from build123d import *

# Parameters (mm, degrees)
BOSS_EXTRUDE1_DEPTH = 25.4
CUT_EXTRUDE1_DEPTH  = 26.4


with BuildPart() as part:
    # Sketch1 → Boss-Extrude1 (new body)
    with BuildSketch(Plane.XY):
        Polygon((0, 0), (-6.35, 10.998522628), (-4.516912895, 10.998522628), (0.916543552, 1.5875), (14.958456448, 1.5875), (15.875, 0), align=None)
    extrude(amount=BOSS_EXTRUDE1_DEPTH)

    # Sketch2 → Cut-Extrude1 (cut, through all)
    with BuildSketch(Plane.XY.offset(25.4)):
        Polygon((-6.35, 10.998522628), (-2.79437447, 8.014998557), (-4.516912895, 10.998522628), align=None)
    extrude(amount=-CUT_EXTRUDE1_DEPTH, mode=Mode.SUBTRACT)


solid = part.part
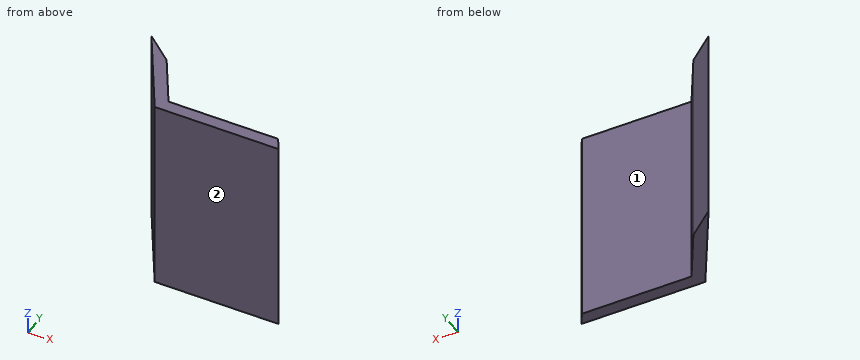
CAD build for the part. Positions are in the model's coordinates, mm. Face numbers are marked on the shaded views. A direction names the side the tool comes from. Give positions to 0.01 mm unless a question says otherwise; leave off trailing zeros. Order: outer loops, then holes, each group sorted by start corner. A loop starts at its lowest first (then second) coordinate and runs counter-clockwise, first axis right, second up. Notation, with made-up numbers: (24, 23) -> (60, 23) arc R15 cw to (60, 45) -> close; hole circle Ø11 at (29.25, 33). An arc over 180 degrees is marked (long way). Return JSON: item names as keys, results as strings.
Q1. Drill centre lines: line 1 (Y direction, x = 12.5, z = 15); line 2 (Y direction, x = -2.5, z = 13); line 3 (X direction, y = 8, z = 20.25). Where is each one in solid material? Low to high.
Working result:
{"line 1": "0 to 1.59", "line 2": "4.33 to 7.51", "line 3": "-4.62 to -2.79"}
Q2. Which spindle directions (+Z, -Z, +X, -X, +Y, -Y) get a long thin tool onto all of the face, cutting with end or side? Do the marked faces 1 and 2. Say none if no direction does.
Working result:
{"face 1": "+Z, -Z, +X, +Y", "face 2": "+Z, -Z, +X, -X, -Y"}
Q3. Flat gauge pins, fed straight in: pin 1 (3 mm diameter, centred on x = 8, z = 14, fed in from +Y); pin 2 (4 mm diameter, centred on y = 2, z = 21.5, fed in from -X); pin 3 (12 mm diameter, centred on x = 1.5, z = 6.5, fed in from +Y). Where does each tip first touch, or does it go through?
Working result:
{"pin 1": "y = 1.59", "pin 2": "x = -2.31", "pin 3": "y = 9.45"}
Q4. Saw through at C-C (y = 6). Write the cut outline in (x, z).
Working result:
{"outline": "(-3.46, 0) -> (-1.63, 0) -> (-1.63, 25.4) -> (-3.46, 25.4) -> close"}
Q5. Saw through at B-B (x = 6.25). Write the cut outline in (y, z), then the cut area to 3 significant figures.
Working result:
{"outline": "(0, 0) -> (1.59, 0) -> (1.59, 25.4) -> (0, 25.4) -> close", "area": "40.3 mm²"}
